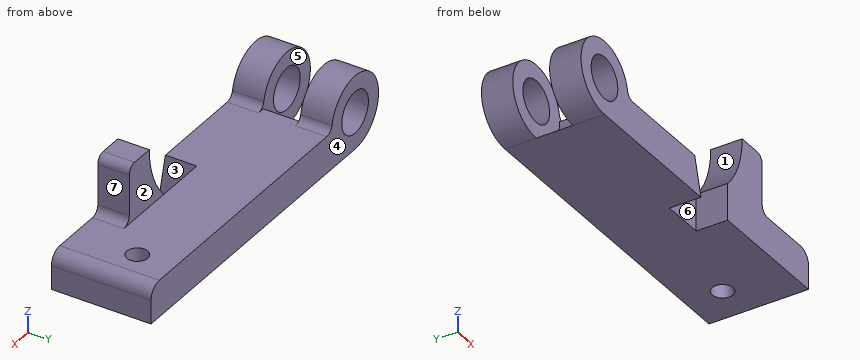
from build123d import *

# Parameters (mm, degrees)
F0_R     = 12.7
F1_DEPTH = 30.1625
F2_DEPTH = 11.1633
F4_DEPTH = 19.05
F5_DEPTH = 19.05
F6_R     = 6.35
F7_DEPTH = 22.353
F8_R     = 7.874
F9_R     = 5.08
F10_R    = 5.08


with BuildPart() as f1:
    # F0 (on Front) → F1 (new body, symmetric)
    with BuildSketch(Plane.XZ):
        with BuildLine():
            ThreePointArc((0, -22.352), (15.8052507731, -15.8052507731), (22.352, 0))
            ThreePointArc((22.352, 0), (-15.8052507731, 15.8052507731), (0, -22.352))
        make_face()
        Circle(F0_R, mode=Mode.SUBTRACT)
        with BuildLine():
            Line((85.852, 0), (22.352, 0))
            ThreePointArc((22.352, 0), (15.8052507731, -15.8052507731), (0, -22.352))
            Line((0, -22.352), (91.8464, -22.352))
            Line((91.8464, -22.352), (85.852, 0))
        make_face()
        Polygon((117.2464, 0), (85.852, 0), (91.8464, -22.352), (117.2464, -22.352), align=None)
        Polygon((150.0886, 0), (117.2464, 0), (117.2464, -22.352), (194.2084, -22.352), (194.2084, 0), align=None)
    extrude(amount=F1_DEPTH, both=True)

    # F0 (on Front) → F2 (cut, symmetric)
    with BuildSketch(Plane.XZ):
        with BuildLine():
            ThreePointArc((0, -22.352), (15.8052507731, -15.8052507731), (22.352, 0))
            ThreePointArc((22.352, 0), (-15.8052507731, 15.8052507731), (0, -22.352))
        make_face()
        Circle(F0_R, mode=Mode.SUBTRACT)
    extrude(amount=F2_DEPTH, both=True, mode=Mode.SUBTRACT)

    # F3 (on face) → F4 (cut)
    with BuildSketch(Plane.XZ.offset(30.1625)):
        Polygon((117.2464, 0), (85.852, 0), (91.8464, -22.352), (117.2464, -22.352), align=None)
    extrude(amount=-F4_DEPTH, mode=Mode.SUBTRACT)

    # F3 (on face) → F5 (join)
    with BuildSketch(Plane.XZ.offset(30.1625)):
        with BuildLine():
            ThreePointArc((131.0386, 34.798), (127.4644153616, 16.0823576341), (117.2464, 0))
            Line((117.2464, 0), (150.0886, 0))
            Line((150.0886, 0), (150.0886, 34.798))
            Line((150.0886, 34.798), (131.0386, 34.798))
        make_face()
    extrude(amount=-F5_DEPTH)

    # F6 (on face) → F7 (cut, through all)
    with BuildSketch(Plane.XY):
        with Locations((172.1485, 7.8105)):
            Circle(F6_R)
    extrude(amount=-F7_DEPTH, mode=Mode.SUBTRACT)

    # F8
    f8_edges = [f1.edges().sort_by_distance(p)[0] for p in [
        (194.2084, 0, 0),
    ]]
    fillet(f8_edges, radius=F8_R)

    # F9
    f9_edges = [f1.edges().sort_by_distance(p)[0] for p in [
        (150.0886, -20.6375, 34.798),
    ]]
    fillet(f9_edges, radius=F9_R)

    # F10
    f10_edges = [f1.edges().sort_by_distance(p)[0] for p in [
        (22.352, -20.6629, 0),
        (22.352, 20.6629, 0),
        (150.0886, -20.6375, 0),
    ]]
    fillet(f10_edges, radius=F10_R)


solid = f1.part
Here's how the part is built. I have some questions about the finished solid (model axes, mm). Face numbers are marked on the shaded views. A direction names the side the tool comes from. Round coordinates to 2 decimals unless told otherwise and drop trailing zeros. Loops run counter-clockwise (first coordinate to the right, second up) from the corner with the lowest first, then second, coordinate; pieces in that order, holes last.
1. If we section it at D-D on x = 39.5: Write out the boundary of the cut face in (y, z), plus the area to 3 significant figures.
Answer list:
outline: (-30.16, -22.35) - (30.16, -22.35) - (30.16, 0) - (-30.16, 0) - close
area: 1,350 mm2
2. We'd pull the mould along Y, two halves only. Please class the marked faces 4, 5, 6 and 7: +Y half, -Y half, draft (parallel to the pull), parting line (faces both ways), or undercut.
Answer list:
face 4: +Y half
face 5: undercut
face 6: -Y half
face 7: draft
3. If we section it at B-B on y = 17: Write out the boundary of the cut face in (x, z), plus the area to 3 significant figures.
Answer list:
outline: (0, -22.35) - (194.21, -22.35) - (194.21, -7.87) arc R7.87 ccw to (186.33, 0) - (26.96, 0) arc R5.08 cw to (21.97, 4.14) arc R22.35 ccw (long way) to start; hole circle Ø25.4 at (0, 0)
area: 5,000 mm2
4. If we section it at A-A on z = -4: Write out the boundary of the cut face in (x, y).
Answer list:
outline: (-21.99, -30.16) - (-12.05, -30.16) - (-12.05, -11.16) - (-21.99, -11.16) - close; (-21.99, 11.16) - (-12.05, 11.16) - (-12.05, 30.16) - (-21.99, 30.16) - close; (12.05, -30.16) - (86.92, -30.16) - (86.92, -11.11) - (117.25, -11.11) - (117.25, -30.16) - (193.19, -30.16) - (193.19, 30.16) - (12.05, 30.16) - (12.05, 11.16) - (21.99, 11.16) - (21.99, -11.16) - (12.05, -11.16) - close; hole circle Ø12.7 at (172.15, 7.81)
5. Which directions (+Z, -Z, +X, -X, +Y, -Y) give clear straight access to the entire face, cutting with the end or side of a thin tool? Please do the marked faces 1, 2 and 3.
Answer list:
face 1: +Z, +Y, -Y
face 2: +Z, +X, -X, +Y
face 3: +Z, -Y
6. For P1, Ø1, axis at x = 76.5, y = -15.5, coming from the +Z side; P2, Ø6.5, axis at x = 95.5, z = -12.5, coming from the -Y side; P3, Ø15, axis at y = -24.5, z = 16.5, coming from the +X side, each with a flat end and sliding along its axis, tell me the tip position at first contact or that it passes through.
Answer list:
P1: stops at z = 0
P2: stops at y = -11.11
P3: stops at x = 150.09
7. If we section it at C-C on z = 10: Write out the boundary of the cut face in (x, y), plus the area to 3 significant figures.
Answer list:
outline: (-19.99, -30.16) - (-7.83, -30.16) - (-7.83, -11.16) - (-19.99, -11.16) - close; (-19.99, 11.16) - (-7.83, 11.16) - (-7.83, 30.16) - (-19.99, 30.16) - close; (7.83, -30.16) - (19.99, -30.16) - (19.99, -11.16) - (7.83, -11.16) - close; (7.83, 11.16) - (19.99, 11.16) - (19.99, 30.16) - (7.83, 30.16) - close; (124.57, -30.16) - (150.09, -30.16) - (150.09, -11.11) - (124.57, -11.11) - close
area: 1,410 mm2
8. If I drill on line 1 along Z through (x, y) = (0, 19); line 2 along Y through (x, z) = (130, 15); line 3 along Z through (x, y) = (127, 11.5), over which ranges is the centre line in solid material (lowest first)?
Answer list:
line 1: z = -22.35 to -12.7, 12.7 to 22.35
line 2: y = -30.16 to -11.11
line 3: z = -22.35 to 0
